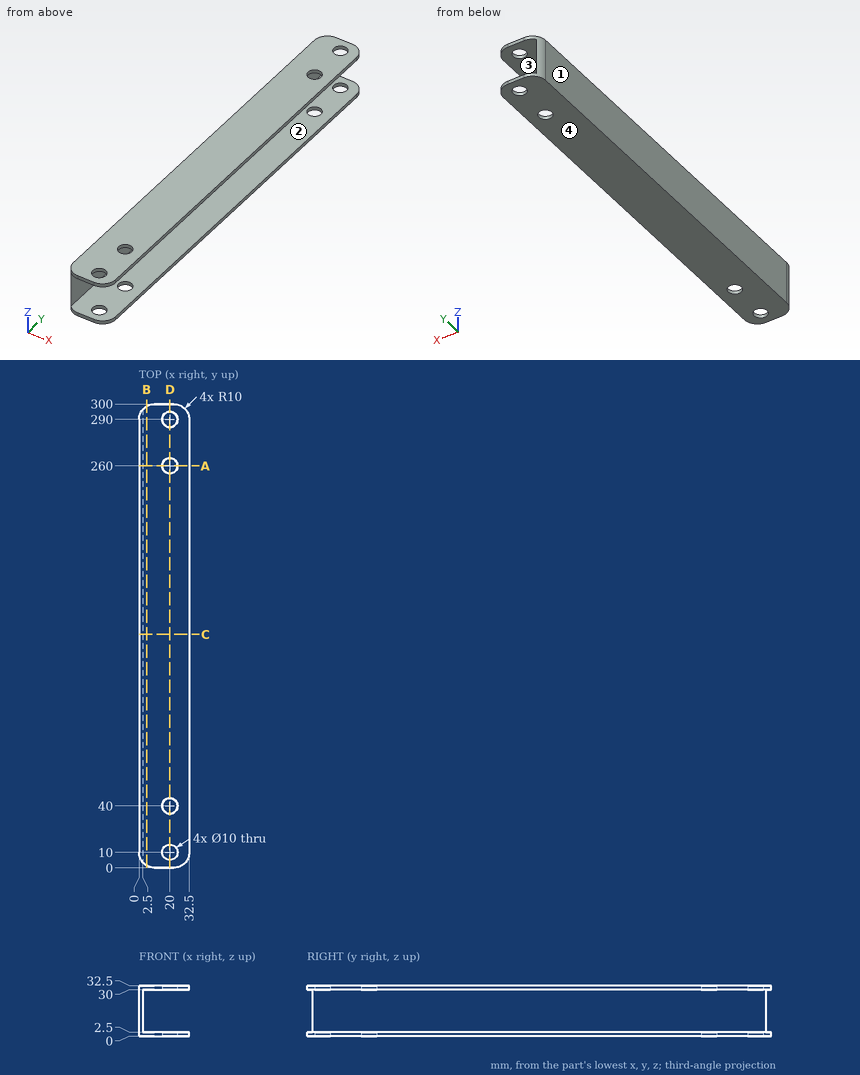
Study the drawing (mm; zero at the part's minimum x, y, z) and answer. Round coordinates to 2 decimals unless told otherwise and drop trailing zeros. Loops run counter-clockwise (first coordinate to the right, second up) from the corner with the lowest first, then second, coordinate; pieces in that order, holes last. Notation, with made-up numbers: (73.5, -39.75) -> (119.5, -39.75) arc R13 ccw to (119.5, -14.75) -> close; hole circle Ø3 at (-10, 23). An arc over 180 degrees is marked (long way). Write each question's results on one line, items separated by ' | '. Start each with the question number.
1. Section C-C (y = 151) is taken. Determine the outline of the cut face in (x, z), plus the area to 3 significant figures.
2. Given pin 1 Ø8 at (y, z) = (122.5, 12) entering from +X; pin 2 Ø8 at (x, y) = (20, 260) entering from +Z, each flat-ended and moving along its own axis, determine where each tip first touches the part or whether it passes through.
3. For a pull along Z with two mould halves and no side action, classify the marked faces 1, 2, 3 and 4 as +Z half, -Z half, draft (parallel to the pull), parting line (faces both ways), or undercut.
4. Section A-A (y = 260) is taken. Determine the outline of the cut face in (x, z), plus the area to 3 significant figures.
5. Section D-D (x = 20) is taken. State how many separate pieces and enclosed holes the cut face has, plus the area to 3 significant figures.
6. Section B-B (x = 5) is taken. Determine the outline of the cut face in (y, z), plus the area to 3 significant figures.
7. Find the intervals of material crossed by probe 1 along Z at (x, y) = (3.5, 23.5); probe 2 along Y at (x, z) = (20, 1.1); probe 3 along X at (y, z) = (290, 1.15), in increasing order. Write a range as from..to.
Evaluation:
1) outline: (0, 0) -> (32.5, 0) -> (32.5, 2.5) -> (2.5, 2.5) -> (2.5, 30) -> (32.5, 30) -> (32.5, 32.5) -> (0, 32.5) -> close | area: 231 mm2
2) pin 1: stops at x = 2.5 | pin 2: passes through
3) face 1: draft | face 2: undercut | face 3: undercut | face 4: -Z half
4) outline: (0, 0) -> (15, 0) -> (15, 2.5) -> (2.5, 2.5) -> (2.5, 30) -> (15, 30) -> (15, 32.5) -> (0, 32.5) -> close; (25, 0) -> (32.5, 0) -> (32.5, 2.5) -> (25, 2.5) -> close; (25, 30) -> (32.5, 30) -> (32.5, 32.5) -> (25, 32.5) -> close | area: 181 mm2
5) separate pieces: 10 | enclosed holes: 0 | area: 1,300 mm2
6) outline: (1.34, 0) -> (298.66, 0) -> (298.66, 2.5) -> (1.34, 2.5) -> close; (1.34, 30) -> (298.66, 30) -> (298.66, 32.5) -> (1.34, 32.5) -> close | area: 1,490 mm2
7) probe 1: z = 0..2.5, 30..32.5 | probe 2: y = 0..5, 15..35, 45..255, 265..285, 295..300 | probe 3: x = 0..15, 25..32.5
